```python
from build123d import *

# Parameters (mm, degrees)
SKETCH1_W               = 38
SKETCH1_H               = 27.5
BOSS_EXTRUDE1_DEPTH     = 6
SKETCH2_W               = 36.5
SKETCH2_H               = 26
CUT_EXTRUDE1_DEPTH      = 2
SKETCH3_RX              = 16.007748615
SKETCH3_RY              = 10.755206101
CUT_EXTRUDE2_DEPTH      = 3
CUT_EXTRUDE2_DEPTH_BACK = 5
CUT_EXTRUDE4_DEPTH      = 1.5
CUT_EXTRUDE5_DEPTH      = 14.7500001
CUT_EXTRUDE5_DEPTH_BACK = 14.7500001


with BuildPart() as part:
    # Sketch1 → Boss-Extrude1 (new body)
    with BuildSketch(Plane(origin=(0, 0, 0), x_dir=(1, 0, 0), z_dir=(0, 1, 0))):
        Rectangle(SKETCH1_W, SKETCH1_H)
    extrude(amount=-BOSS_EXTRUDE1_DEPTH)

    # Sketch2 → Cut-Extrude1 (cut)
    with BuildSketch(Plane(origin=(0, 0, 0), x_dir=(1, 0, 0), z_dir=(0, 1, 0))):
        Rectangle(SKETCH2_W, SKETCH2_H)
    extrude(amount=-CUT_EXTRUDE1_DEPTH, mode=Mode.SUBTRACT)

    # Sketch3 → Cut-Extrude2 (cut, two sides)
    with BuildSketch(Plane(origin=(0, -2, 0), x_dir=(1, 0, 0), z_dir=(0, 1, 0))) as cut_extrude2_sk:
        with Locations(Location((0, 0), (0, 0, -1.782797699))):
            Ellipse(SKETCH3_RX, SKETCH3_RY)
    extrude(amount=CUT_EXTRUDE2_DEPTH, mode=Mode.SUBTRACT)
    extrude(cut_extrude2_sk.sketch, amount=-CUT_EXTRUDE2_DEPTH_BACK, mode=Mode.SUBTRACT)

    # Sketch8 → Cut-Extrude4 (cut, symmetric)
    with BuildSketch(Plane(origin=(0, -4, 0), x_dir=(-1, 0, 0), z_dir=(0, -1, 0))):
        with BuildLine():
            Line((-14.5, 11), (-14.5, 23.562662058))
            Line((-14.5, 23.562662058), (-9.5, 23.562662058))
            Line((-9.5, 23.562662058), (-9.5, 11))
            ThreePointArc((-9.5, 11), (-12, 8.5), (-14.5, 11))
        make_face()
        with BuildLine():
            Line((9.5, 23.562662058), (9.5, 11))
            ThreePointArc((9.5, 11), (12, 8.5), (14.5, 11))
            Line((14.5, 11), (14.5, 23.562662058))
            Line((14.5, 23.562662058), (9.5, 23.562662058))
        make_face()
        with BuildLine():
            Line((14.5, -11), (14.5, -23.562662058))
            Line((14.5, -23.562662058), (9.5, -23.562662058))
            Line((9.5, -23.562662058), (9.5, -11))
            ThreePointArc((9.5, -11), (12, -8.5), (14.5, -11))
        make_face()
        with BuildLine():
            Line((-9.5, -23.562662058), (-9.5, -11))
            ThreePointArc((-9.5, -11), (-12, -8.5), (-14.5, -11))
            Line((-14.5, -11), (-14.5, -23.562662058))
            Line((-14.5, -23.562662058), (-9.5, -23.562662058))
        make_face()
    extrude(amount=CUT_EXTRUDE4_DEPTH, both=True, mode=Mode.SUBTRACT)

    # Sketch9 → Cut-Extrude5 (cut, two sides)
    with BuildSketch(Plane.XY) as cut_extrude5_sk:
        Polygon((-19, -2), (-16.199169847, -6), (-19, -6), align=None)
        Polygon((16.199169847, -6), (19, -6), (19, -2), align=None)
    extrude(amount=CUT_EXTRUDE5_DEPTH, mode=Mode.SUBTRACT)
    extrude(cut_extrude5_sk.sketch, amount=-CUT_EXTRUDE5_DEPTH_BACK, mode=Mode.SUBTRACT)


solid = part.part
```
Design review of the part built by this model. Coordinates are the model's own, in mm. A direction names the side the tool comes from. Coordinates: 2 decimals unless noted, no trailing zeros. Use CSV: the item, a comma, the result in double quotes. Start each with the question number.
1) Tool access review of faces 1 (the flat face through (0, -1, -13)), 2 (the flat face through (0, -3, 13.75)), 3 (the flat face through (-14.5, -4, -12)), 4 (the flat face through (-14.5, -4, 12)): name each direction out of +Z, -Z, +X, -X, +Y, -Y from which nothing blocks a thin tool from reaching the whole face with its end or side.
2) Wall thickness on L1, parallel to Z at x = 10.5, y = -1.5; L2, parallel to X at y = -3.25, z = -9; L3, parallel to X at y = -0.25, z = 2: over which ranges is each line inside the solid? List them lowest first. Write a range as from..to.
3) Consider section A-A on z = 9.5. Give the number of separate pieces and of enclosed holes in the cut face, then the cut area to 3 significant figures.
4) The part is to be moulded in two halves that separate along X. For faces 5 (the flat face through (-12, -5.5, -11)), 6 (the flat face through (0, -3, -13.75)), say which applies: +X half, -X half, draft (parallel to the pull), parting line (faces both ways), or undercut.
5) For pin 1 Ø0.8 at (y, z) = (-4, 12.5) entering from -X; pin 2 Ø0.8 at (y, z) = (-3.5, 12) entering from +X; pin 3 Ø0.8 at (y, z) = (-4.5, -12) entering from +X; pin 4 Ø2.5 at (x, z) = (-11, 12) entering from +Y, all flat-tipped, find the tip position at first contact; note any pin that passes through.
Geometry says:
1,face 1,"+Y"
1,face 2,"+Z, +X, -X, +Y, -Y"
1,face 3,"-Z"
1,face 4,"+Z"
2,L1,"-13.75..-13, 13..13.75"
2,L2,"-18.12..-13.5, -10.5..-9.11, 8.43..10.5, 13.5..18.12"
2,L3,"-19..-18.25, 18.25..19"
3,separate pieces,"2"
3,enclosed holes,"2"
3,area,"59.7 mm^2"
4,face 5,"undercut"
4,face 6,"draft"
5,pin 1,"x = -17.88"
5,pin 2,"x = 18.23"
5,pin 3,"x = 17.53"
5,pin 4,"y = 0"
